For this review, take the finished solid that the model builds, in its own axes (mm). Face numbers are marked on the shaded views. A direction names the side the tool comes from. Round coordinates to 2 decimals unless told otherwise and drop trailing zeros. Order: outer loops, then holes, each group sorted by start corner. A loop starts at its lowest first (then second) coordinate and runs counter-clockwise, first axis right, second up. Notation, with made-up numbers: (-31, -26.5) -> (-22, -26.5) arc R15 ccw to (-22, -18.5) -> close; hole circle Ø8 at (6.5, -27). An arc over 180 degrees is marked (long way). Use a Markdown table: item, result. Add a question column.
1) Draft analysis for pull direction X (two halves, no side actions). For the marked faces 6, 7 and 8, state which applies: pulls with the +X half, pulls with the -X half, needs draft (parallel to the pull), parting line crosses it, or undercut.
2) Consider section D-D (z = 71.5). State the section outline as (x, y) points, plus the area to 3 significant figures.
3) Consider section B-B (z = 41.5). State the section outline as (x, y) points (3 decimals), plus the area to 3 significant figures.
4) Consider section A-A (z = -17). State the section outline as (x, y) points (3 decimals), plus the area to 3 significant figures.
5) Machinability: for the marked faces 1, 2, 3, 4 and 5, which of the approach directions +Z, -Z, +X, -X, +Y, -Y give a long, thin tool a straight path to every point of the face, cutting with its end or side? Answer none if there is none.
6) Clearance check with flat-ended pins moving along their axes: P1, Ø22, axis at x = -93.65, y = 0, coming from the -Z side; P2, Ø5, axis at x = -49.15, y = 15.5, coming from the -Z side; P3, Ø8, axis at y = 7, z = -9, coming from the -X side (3 decimals). State where each tip first meets the part, or that it passes through.
7) Wall thickness on line 1 along X through (y, z) = (-4.5, -0.5) (3 decimals); line 2 along Y through (x, z) = (-64.65, 79.5); line 3 along X through (y, z) = (0, 11.5): over which ranges is each line inside the solid? List them lowest first. Write a range as [from, to].
8) Consider section C-C (x = -7). State the section outline as (y, z) points, plus the area to 3 significant figures.
```python
from build123d import *

# Parameters (mm, degrees)
SKETCH5_R       = 9.46
SKETCH5_R_2     = 1.6
EXTRUDE1_DEPTH  = 5
SKETCH6_R       = 9.46
EXTRUDE2_DEPTH  = 40
SKETCH7_W       = 49.45
SKETCH7_H       = 49.45
SKETCH7_W_2     = 43.1
SKETCH7_H_2     = 43.1
EXTRUDE3_DEPTH  = 35
EXTRUDE5_REACH  = 20.597
EXTRUDE6_REACH  = 20.597
SKETCH16_R      = 7
EXTRUDE9_DEPTH  = 49.45
EXTRUDE10_DEPTH = 17
SKETCH18_R      = 12.7
SKETCH18_R_2    = 9.46
EXTRUDE11_DEPTH = 14
SKETCH19_R      = 11.1
SKETCH19_R_2    = 9.46
EXTRUDE12_DEPTH = 7
SKETCH20_R      = 9.46
SKETCH20_R_2    = 9.2
EXTRUDE13_DEPTH = 3
EXTRUDE14_DEPTH = 15
SKETCH22_R      = 3.2
EXTRUDE15_DEPTH = 3
SKETCH23_R      = 3.2
EXTRUDE16_DEPTH = 3
SKETCH24_R      = 7
EXTRUDE17_DEPTH = 49.45
SKETCH25_R      = 6.5
EXTRUDE18_DEPTH = 5
EXTRUDE19_START = -25.300694
SKETCH26_R      = 1.5
EXTRUDE19_DEPTH = 119.050001


with BuildPart() as part:
    # Sketch5 → Extrude1 (new body)
    with BuildSketch(Plane.XY):
        with BuildLine():
            Line((-21.825, -24.725), (0, -12.7))
            ThreePointArc((0, -12.7), (12.7, 0), (0, 12.7))
            Line((0, 12.7), (-21.825, 24.725))
            Line((-21.825, 24.725), (-89.375, 24.725))
            Line((-89.375, 24.725), (-93.65, 12.7))
            ThreePointArc((-93.65, 12.7), (-106.35, 0), (-93.65, -12.7))
            Line((-93.65, -12.7), (-89.375, -24.725))
            Line((-89.375, -24.725), (-21.825, -24.725))
        make_face()
        Circle(SKETCH5_R, mode=Mode.SUBTRACT)
        with Locations((-93.65, 0)):
            Circle(SKETCH5_R, mode=Mode.SUBTRACT)
        with Locations((-31.05, 15.5)):
            Circle(SKETCH5_R_2, mode=Mode.SUBTRACT)
        with Locations((-31.05, -15.5)):
            Circle(SKETCH5_R_2, mode=Mode.SUBTRACT)
        with Locations((-49.15, -15.5)):
            Circle(SKETCH5_R_2, mode=Mode.SUBTRACT)
        with Locations((-49.15, 15.5)):
            Circle(SKETCH5_R_2, mode=Mode.SUBTRACT)
        with Locations((-62.05, 15.5)):
            Circle(SKETCH5_R_2, mode=Mode.SUBTRACT)
        with Locations((-80.15, 15.5)):
            Circle(SKETCH5_R_2, mode=Mode.SUBTRACT)
        with Locations((-80.15, -15.5)):
            Circle(SKETCH5_R_2, mode=Mode.SUBTRACT)
        with Locations((-62.05, -15.5)):
            Circle(SKETCH5_R_2, mode=Mode.SUBTRACT)
    extrude(amount=EXTRUDE1_DEPTH)

    # Sketch6 → Extrude2 (add)
    with BuildSketch(Plane.XY.offset(5)):
        with BuildLine():
            Line((-39.925, 24.725), (-89.375, 24.725))
            Line((-89.375, 24.725), (-93.65, 12.7))
            ThreePointArc((-93.65, 12.7), (-106.35, 0), (-93.65, -12.7))
            Line((-93.65, -12.7), (-89.375, -24.725))
            Line((-89.375, -24.725), (-39.925, -24.725))
            Line((-39.925, -24.725), (-39.925, -1.585093616))
            Line((-39.925, -1.585093616), (-12.600693561, -1.585093616))
            ThreePointArc((-12.600693561, -1.585093616), (-9.51301391, -8.413831847), (-3.112651943, -12.312651943))
            Line((-3.112651943, -12.312651943), (-25, -24.725))
            Line((-25, -24.725), (-21.825, -24.725))
            Line((-21.825, -24.725), (0, -12.7))
            ThreePointArc((0, -12.7), (12.7, 0), (0, 12.7))
            Line((0, 12.7), (-21.825, 24.725))
            Line((-21.825, 24.725), (-25, 24.725))
            Line((-25, 24.725), (-3.112651943, 12.312651943))
            ThreePointArc((-3.112651943, 12.312651943), (-9.513885465, 8.41284633), (-12.601021697, 1.58248292))
            Line((-12.601021697, 1.58248292), (-39.925, 1.58248292))
            Line((-39.925, 1.58248292), (-39.925, 24.725))
        make_face()
        Circle(SKETCH6_R, mode=Mode.SUBTRACT)
        with BuildLine():
            Line((-86.2, -21.55), (-43.1, -21.55))
            Line((-43.1, -21.55), (-43.1, 21.55))
            Line((-43.1, 21.55), (-86.2, 21.55))
            Line((-86.2, 21.55), (-86.2, 15.891608363))
            ThreePointArc((-86.2, 15.891608363), (-89.375, 12.716608363), (-86.2, 9.541608363))
            Line((-86.2, 9.541608363), (-86.2, 5.830017153))
            ThreePointArc((-86.2, 5.830017153), (-103.11, 0), (-86.2, -5.830017153))
            Line((-86.2, -5.830017153), (-86.2, -9.508391637))
            ThreePointArc((-86.2, -9.508391637), (-89.375, -12.683391637), (-86.2, -15.858391637))
            Line((-86.2, -15.858391637), (-86.2, -21.55))
        make_face(mode=Mode.SUBTRACT)
    extrude(amount=EXTRUDE2_DEPTH)

    # Sketch7 → Extrude3 (add)
    with BuildSketch(Plane(origin=(0, 0, 0), x_dir=(-1, 0, 0), z_dir=(0, 0, -1))):
        with Locations((46.55, 0)):
            Rectangle(SKETCH7_W, SKETCH7_H)
        with Locations((46.55, 0)):
            Rectangle(SKETCH7_W_2, SKETCH7_H_2, mode=Mode.SUBTRACT)
    extrude(amount=EXTRUDE3_DEPTH)

    # Extrude5: up to this face of the body (flat: up to its plane)
    extrude5_end = Plane(part.part.faces().sort_by_distance((-10.9125, 18.7125, 22.5))[0])
    # Sketch12 → Extrude5 (cut, up to the picked face)
    with BuildSketch(Plane(origin=(4.5259255, 7.980803168, 0), x_dir=(0, 0, 1), z_dir=(-0.493298857, -0.869859895, 0)), mode=Mode.PRIVATE) as extrude5_sk1:
        Polygon((45, 8.781388226), (5, 33.943311626), (45, 33.943311626), align=None)
    extrude5_tool1 = split(extrude(extrude5_sk1.sketch, amount=-EXTRUDE5_REACH, mode=Mode.PRIVATE), bisect_by=extrude5_end, keep=Keep.BOTH, mode=Mode.PRIVATE)
    add(extrude5_tool1.solids().sort_by_distance((-17.704217, 20.587551, 31.666667))[0], mode=Mode.SUBTRACT)

    # Extrude6: up to this face of the body (flat: up to its plane)
    extrude6_end = Plane(part.part.faces().sort_by_distance((-10.9125, -18.7125, 22.5))[0])
    # Sketch13 → Extrude6 (cut, up to the picked face)
    with BuildSketch(Plane(origin=(4.5259255, -7.980803168, 0), x_dir=(0, 0, 1), z_dir=(-0.493298857, 0.869859895, 0)), mode=Mode.PRIVATE) as extrude6_sk1:
        Polygon((45, -8.781388226), (5, -33.943311626), (45, -33.943311626), align=None)
    extrude6_tool1 = split(extrude(extrude6_sk1.sketch, amount=-EXTRUDE6_REACH, mode=Mode.PRIVATE), bisect_by=extrude6_end, keep=Keep.BOTH, mode=Mode.PRIVATE)
    add(extrude6_tool1.solids().sort_by_distance((-17.704217, -20.587551, 31.666667))[0], mode=Mode.SUBTRACT)

    # Sketch16 → Extrude9 (cut)
    with BuildSketch(Plane.XZ.offset(24.725)):
        with Locations((-46.55, -17)):
            Circle(SKETCH16_R)
        with Locations((-67.618096531, 17)):
            Circle(SKETCH16_R)
        Polygon((-39.925, 22), (-16.781973348, 22.403360483), (-12.600693561, 29.053940018), (-12.600693561, 45), (-86.2, 45), (-54.981583076, 22), align=None)
    extrude(amount=-EXTRUDE9_DEPTH, mode=Mode.SUBTRACT)

    # Sketch17 → Extrude10 (add)
    with BuildSketch(Plane.XY.offset(45)):
        with BuildLine():
            Line((-86.2, 10.285305051), (-86.2, 5.830017153))
            ThreePointArc((-86.2, 5.830017153), (-103.11, 0), (-86.2, -5.830017153))
            Line((-86.2, -5.830017153), (-86.2, -10.285305051))
            ThreePointArc((-86.2, -10.285305051), (-89.146529591, -11.874710703), (-92.40601106, -12.638927625))
            ThreePointArc((-92.40601106, -12.638927625), (-106.334722718, -0.62274359), (-93.65, 12.7))
            ThreePointArc((-93.65, 12.7), (-89.734222565, 12.081253539), (-86.2, 10.285305051))
        make_face()
    extrude(amount=EXTRUDE10_DEPTH)

    # Sketch18 → Extrude11 (add)
    with BuildSketch(Plane.XY.offset(62)):
        with Locations((-93.65, 0)):
            Circle(SKETCH18_R)
        with Locations((-93.65, 0)):
            Circle(SKETCH18_R_2, mode=Mode.SUBTRACT)
    extrude(amount=EXTRUDE11_DEPTH)

    # Sketch19 → Extrude12 (add)
    with BuildSketch(Plane.XY.offset(76)):
        with BuildLine():
            Line((-81.398348387, -6.344577353), (-76.315821236, -6.344577353))
            ThreePointArc((-76.315821236, -6.344577353), (-51.370502761, 0), (-76.315821236, 6.344577353))
            Line((-76.315821236, 6.344577353), (-81.398348387, 6.344577353))
            ThreePointArc((-81.398348387, 6.344577353), (-107.446978982, 0), (-81.398348387, -6.344577353))
        make_face()
        with Locations((-64.65, 0)):
            Circle(SKETCH19_R, mode=Mode.SUBTRACT)
        with Locations((-93.65, 0)):
            Circle(SKETCH19_R_2, mode=Mode.SUBTRACT)
    extrude(amount=EXTRUDE12_DEPTH)

    # Sketch20 → Extrude13 (add)
    with BuildSketch(Plane.XY.offset(83)):
        with BuildLine():
            Line((-81.398348387, -6.344577353), (-76.315821236, -6.344577353))
            ThreePointArc((-76.315821236, -6.344577353), (-51.370502761, 0), (-76.315821236, 6.344577353))
            Line((-76.315821236, 6.344577353), (-81.398348387, 6.344577353))
            ThreePointArc((-81.398348387, 6.344577353), (-107.446978982, 0), (-81.398348387, -6.344577353))
        make_face()
        with Locations((-93.65, 0)):
            Circle(SKETCH20_R, mode=Mode.SUBTRACT)
        with Locations((-64.65, 0)):
            Circle(SKETCH20_R_2, mode=Mode.SUBTRACT)
    extrude(amount=EXTRUDE13_DEPTH)

    # Sketch21 → Extrude14 (cut)
    with BuildSketch(Plane.ZY.offset(43.1)):
        Polygon((76, 0), (76, -2.7), (83, -2.7), (83, 2.7), (76, 2.7), align=None)
    extrude(amount=EXTRUDE14_DEPTH, mode=Mode.SUBTRACT)

    # Sketch22 → Extrude15 (cut)
    with BuildSketch(Plane.XY.offset(5)):
        with Locations((-62.05, 15.5)):
            Circle(SKETCH22_R)
        with Locations((-62.05, -15.5)):
            Circle(SKETCH22_R)
    extrude(amount=-EXTRUDE15_DEPTH, mode=Mode.SUBTRACT)

    # Sketch23 → Extrude16 (cut)
    with BuildSketch(Plane(origin=(0, 0, 0), x_dir=(-1, 0, 0), z_dir=(0, 0, -1))):
        with Locations((49.15, 15.5)):
            Circle(SKETCH23_R)
        with Locations((49.15, -15.5)):
            Circle(SKETCH23_R)
    extrude(amount=-EXTRUDE16_DEPTH, mode=Mode.SUBTRACT)

    # Sketch24 → Extrude17 (cut)
    with BuildSketch(Plane.ZY.offset(71.275)):
        with Locations((-17, 0)):
            Circle(SKETCH24_R)
        with BuildLine():
            Line((0, 0), (0, 4))
            ThreePointArc((0, 4), (-4, 0), (0, -4))
            Line((0, -4), (0, 0))
        make_face()
    extrude(amount=-EXTRUDE17_DEPTH, mode=Mode.SUBTRACT)

    # Sketch25 → Extrude18 (cut)
    with BuildSketch(Plane(origin=(0, 0, 0), x_dir=(-1, 0, 0), z_dir=(0, 0, -1))):
        with Locations((46.55, 0)):
            Circle(SKETCH25_R)
        with Locations((64.65, 0)):
            Circle(SKETCH25_R)
    extrude(amount=-EXTRUDE18_DEPTH, mode=Mode.SUBTRACT)

    # Sketch26 → Extrude19 (cut)
    with BuildSketch(Plane.ZY.offset(12.600693561).offset(EXTRUDE19_START)):
        with Locations((30, 0)):
            Circle(SKETCH26_R)
    extrude(amount=EXTRUDE19_DEPTH, mode=Mode.SUBTRACT)


solid = part.part
```
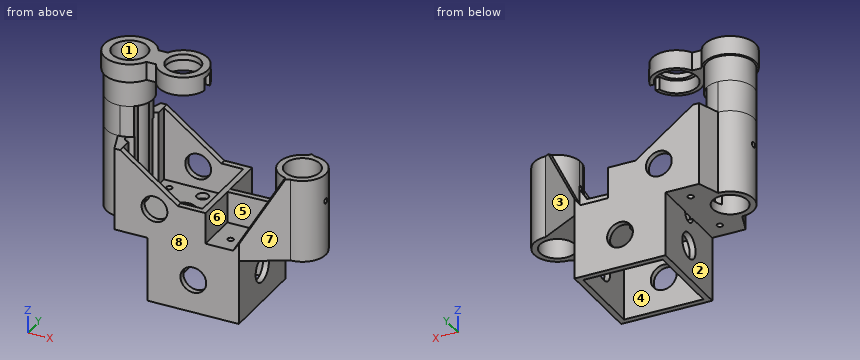
Results list:
| question | item | result |
|---|---|---|
| 1 | face 6 | undercut |
| 1 | face 7 | pulls with the +X half |
| 1 | face 8 | needs draft |
| 2 | outline | circle Ø25.4 at (-93.65, 0); hole circle Ø18.92 at (-93.65, 0) |
| 2 | area | 226 mm2 |
| 3 | outline | (-93.65, -12.7) -> (-89.375, -24.725) -> (-81.449, -24.725) -> (-81.449, -21.55) -> (-86.2, -21.55) -> (-86.2, -15.858) arc R3.175 cw to (-86.2, -9.508) -> (-86.2, -5.83) arc R9.46 cw (long way) to (-86.2, 5.83) -> (-86.2, 9.542) arc R3.175 cw to (-86.2, 15.892) -> (-86.2, 21.55) -> (-81.449, 21.55) -> (-81.449, 24.725) -> (-89.375, 24.725) -> (-93.65, 12.7) arc R12.7 ccw to start; (-12.601, -1.585) arc R12.7 ccw to (-3.113, -12.313) -> (-5.028, -13.399) -> (-4.133, -14.977) -> (0, -12.7) arc R12.7 ccw to (0, 12.7) -> (-4.133, 14.977) -> (-5.028, 13.399) -> (-3.113, 12.313) arc R12.7 ccw to (-12.601, 1.585) -> close; hole circle Ø18.92 at (0, 0) |
| 3 | area | 541 mm2 |
| 4 | outline | (-71.275, -24.725) -> (-53.55, -24.725) -> (-53.55, -21.55) -> (-68.1, -21.55) -> (-68.1, -7) -> (-71.275, -7) -> close; (-71.275, 7) -> (-68.1, 7) -> (-68.1, 21.55) -> (-53.55, 21.55) -> (-53.55, 24.725) -> (-71.275, 24.725) -> close; (-39.55, -24.725) -> (-21.825, -24.725) -> (-21.825, -7) -> (-25, -7) -> (-25, -21.55) -> (-39.55, -21.55) -> close; (-39.55, 21.55) -> (-25, 21.55) -> (-25, 7) -> (-21.825, 7) -> (-21.825, 24.725) -> (-39.55, 24.725) -> close |
| 4 | area | 410 mm2 |
| 5 | face 1 | +Z, -Z |
| 5 | face 2 | -Z, -X, +Y, -Y |
| 5 | face 3 | +Z, -Z, +X, +Y |
| 5 | face 4 | -Z |
| 5 | face 5 | +Z |
| 6 | P1 | z = 0 |
| 6 | P2 | z = 3 |
| 6 | P3 | x = -71.275 |
| 7 | line 1 | [-71.275, -68.1], [-25, -21.825] |
| 7 | line 2 | [-13.28, -11.1], [11.1, 13.28] |
| 7 | line 3 | [-106.35, -103.11], [-43.1, -9.46], [9.46, 12.7] |
| 8 | outline | (-16.56, 0) -> (-6.36, 0) -> (-6.36, 45) -> (-10.6, 45) -> (-10.6, 5) -> (-14.52, 5) -> (-14.52, 37.9) -> (-16.56, 36.3) -> close; (6.36, 0) -> (16.56, 0) -> (16.56, 36.3) -> (14.52, 37.9) -> (14.52, 5) -> (10.6, 5) -> (10.6, 45) -> (6.36, 45) -> close |
| 8 | area | 572 mm2 |
